from build123d import *

# Parameters (mm, degrees)
F1_DEPTH    = 63.5
F0_W        = 25.4
F0_H        = 19.05
F2_DEPTH    = 25.4
F3_DEPTH    = 7.9375
F5_T1_DEPTH = 44.45


# Not quite as in the source:
# - a fillet or chamfer that OpenCascade refuses, or shapes differently, is made with other operations: its cross-section is extruded or revolved along the edge and cut away or added


with BuildPart() as f1:
    # F0 (on Front) → F1 (new body, symmetric)
    with BuildSketch(Plane.XZ):
        Polygon((22.225, 9.525), (-41.275, 9.525), (-41.275, -9.525), (41.275, -9.525), (41.275, 9.525), align=None)
    extrude(amount=F1_DEPTH, both=True)

    # F0 (on Front) → F2 (join, symmetric)
    with BuildSketch(Plane.XZ):
        with BuildLine():
            Line((22.225, 27.0002), (22.225, 9.525))
            Line((22.225, 9.525), (41.275, 9.525))
            Line((41.275, 9.525), (41.275, 27.0002))
            ThreePointArc((41.275, 27.0002), (45.9246798487, 38.2255201513), (57.15, 42.8752))
            Line((57.15, 42.8752), (60.325, 42.8752))
            Line((60.325, 42.8752), (60.325, 61.9252))
            Line((60.325, 61.9252), (57.15, 61.9252))
            add(Edge.make_bspline(
                [(54.3750515166, 61.8147843852), (55.3086427557, 61.8565061807), (56.2339227715, 61.893230908), (57.15, 61.9252)],
                knots=[108.9702028018, 108.9702028018, 108.9702028018, 108.9702028018, 111.5045361635, 111.5045361635, 111.5045361635, 111.5045361635], degree=3))
            ThreePointArc((54.3750515166, 61.8147843852), (31.4919534962, 50.6945089076), (22.225, 27.0002))
        make_face()
        with Locations((73.025, 52.4002)):
            Rectangle(F0_W, F0_H)
    extrude(amount=F2_DEPTH, both=True)

    # F0 (on Front) → F3 (join, symmetric)
    with BuildSketch(Plane.XZ):
        with BuildLine():
            add(Edge.make_bspline(
                [(-41.275, 9.525), (-41.275, 48.9883726548), (14.232887036, 60.0208481258), (54.3750515166, 61.8147843852)],
                knots=[0, 0, 0, 0, 108.9702028018, 108.9702028018, 108.9702028018, 108.9702028018], degree=3))
            Line((-41.275, 9.525), (22.225, 9.525))
            Line((22.225, 9.525), (22.225, 27.0002))
            ThreePointArc((22.225, 27.0002), (31.4919534962, 50.6945089076), (54.3750515166, 61.8147843852))
        make_face()
    extrude(amount=F3_DEPTH, both=True)

    # F0 (on Front) → F4 (revolve)
    with BuildSketch(Plane.XZ):
        Polygon((85.725, 66.675), (85.725, 61.9252), (85.725, 42.8752), (85.725, 38.1), (111.125, 38.1), (111.125, 66.675), align=None)
    revolve(axis=Axis((85.725, 0, 52.3875), (0, 0, 1)))

    # F5: fillet of radius 5.08 on 4 edges, made by hand

    # F5_s2 → F5_t1 (cut)
    with BuildSketch(Plane.XY.offset(-22.225)):
        with BuildLine():
            add(Edge.make_bspline(
                [(41.275, -58.42), (41.275, -63.5), (36.195, -63.5)],
                knots=[0, 0, 0, 1, 1, 1], degree=2, weights=[1, 1, 1]))
            Line((36.195, -63.5), (41.275, -63.5))
            Line((41.275, -63.5), (41.275, -58.42))
        make_face()
        with BuildLine():
            add(Edge.make_bspline(
                [(-41.275, -58.42), (-41.275, -63.5), (-36.195, -63.5)],
                knots=[0, 0, 0, 1, 1, 1], degree=2, weights=[1, 1, 1]))
            Line((-36.195, -63.5), (-41.275, -63.5))
            Line((-41.275, -63.5), (-41.275, -58.42))
        make_face()
        with BuildLine():
            add(Edge.make_bspline(
                [(41.275, 58.42), (41.275, 63.5), (36.195, 63.5)],
                knots=[0, 0, 0, 1, 1, 1], degree=2, weights=[1, 1, 1]))
            Line((36.195, 63.5), (41.275, 63.5))
            Line((41.275, 63.5), (41.275, 58.42))
        make_face()
        with BuildLine():
            add(Edge.make_bspline(
                [(-41.275, 58.42), (-41.275, 63.5), (-36.195, 63.5)],
                knots=[0, 0, 0, 1, 1, 1], degree=2, weights=[1, 1, 1]))
            Line((-36.195, 63.5), (-41.275, 63.5))
            Line((-41.275, 63.5), (-41.275, 58.42))
        make_face()
    extrude(amount=F5_T1_DEPTH, mode=Mode.SUBTRACT)


solid = f1.part
Work out the finished part from the listing and answer in its coordinate system (mm). A direction names the side the tool comes from. Round coordinates to 2 decimals unless told otherwise and drop trailing zeros. Order: outer loops, then holes, each group sorted by start corner. A loop starts at its lowest first (then second) coordinate and runs counter-clockwise, first axis right, second up. Notation, with made-up numbers: M 25,88 L 75,88 A28 ccw 75,106 Z; hole C 83.5,64 d11. An arc over 180 degrees is marked long. One line per item, written item: value.
Q1. Find section A-A on y = 56. Write down the section's boundary in (x, z) (3 decimals), then the cut area to 3 significant figures.
Derived:
outline: M -41.275,-9.525 L 41.275,-9.525 L 41.275,9.525 L -41.275,9.525 Z
area: 1,570 mm²
Q2. Flat-ended cylindrical pins translate along their axes: pin 1 (15 mm diameter, centred on x = 80.5, y = 9, fed in from -Z); pin 2 (12 mm diameter, centred on x = 35, z = 33, fed in from +Y); pin 3 (15.5 mm diameter, centred on x = 64, z = 41, fed in from -Y). Find the tip coordinate at first contact, or state that the pin passes through.
Derived:
pin 1: z = 38.1
pin 2: y = 25.4
pin 3: y = -25.4
Q3. Straight lines are drawn through the part: line 1 (Z direction, x = 80.5, y = 11) (3 decimals); line 2 (Y direction, x = 45, z = 58); line 3 (X direction, y = -14.5, z = 8.5) (3 decimals). For each, find the intervals that lie inside material, in ascending order.
Derived:
line 1: 38.1 to 66.675
line 2: -25.4 to 25.4
line 3: -41.275 to 41.275
Q4. For faces 1 (the face through (60, 2, 42.875)), 2 (the face through (-3, 7.938, 30)), 3 (the face through (60, -2, 61.925)), 4 (the face through (-3, -7.938, 30)), 5 (the face through (46, -25.4, 42)), determine the directions among +Z, -Z, +X, -X, +Y, -Y from which every point of the face is accessible in a straight line to the end or side of a thin tool.
Derived:
face 1: -Z
face 2: +Z, -X, +Y
face 3: +Z, -X
face 4: +Z, -X, -Y
face 5: +Z, +X, -X, -Y
